Part print with two shaded views. Sizes in mm from the minimum x, y, z corner. Coordinates: 2 decimals unless noted, no trailing zeros. Write each loop counter-clockwise with the first axis right and the second up, starting at its lowest first coordinate (ties: lowest second). Pieces come first, ordered by that corner, then holes. Notation, with made-up numbers: (21, 86) - (77, 86) arc R5 cw to (77, 93) - close; hole circle Ø7 at (-27.5, -34). An arc over 180 degrees is marked (long way). Answer in a Markdown table with one row per item. Add a question column.
Q1. Band-saw the part on D-D (z = 20). List the corners of the cut face in (x, y).
Q2. Band-saw the part on C-C (x = 107.5). List the corners of the cut face in (y, z).
Q3. Drill centre lines: line 1 along Z through (x, y) = (205.25, 107.5); line 2 along Y through (x, z) = (104, 67.5). Where is each one in solid material? Low to high. Write a range as from..to.
Q4. Band-saw the part on A-A (y = 107.5). List the corners of the cut face in (x, z), and give its area (4 significant figures).
Q5. Band-saw the part on B-B (z = 106). List the corners of the cut face in (x, y).
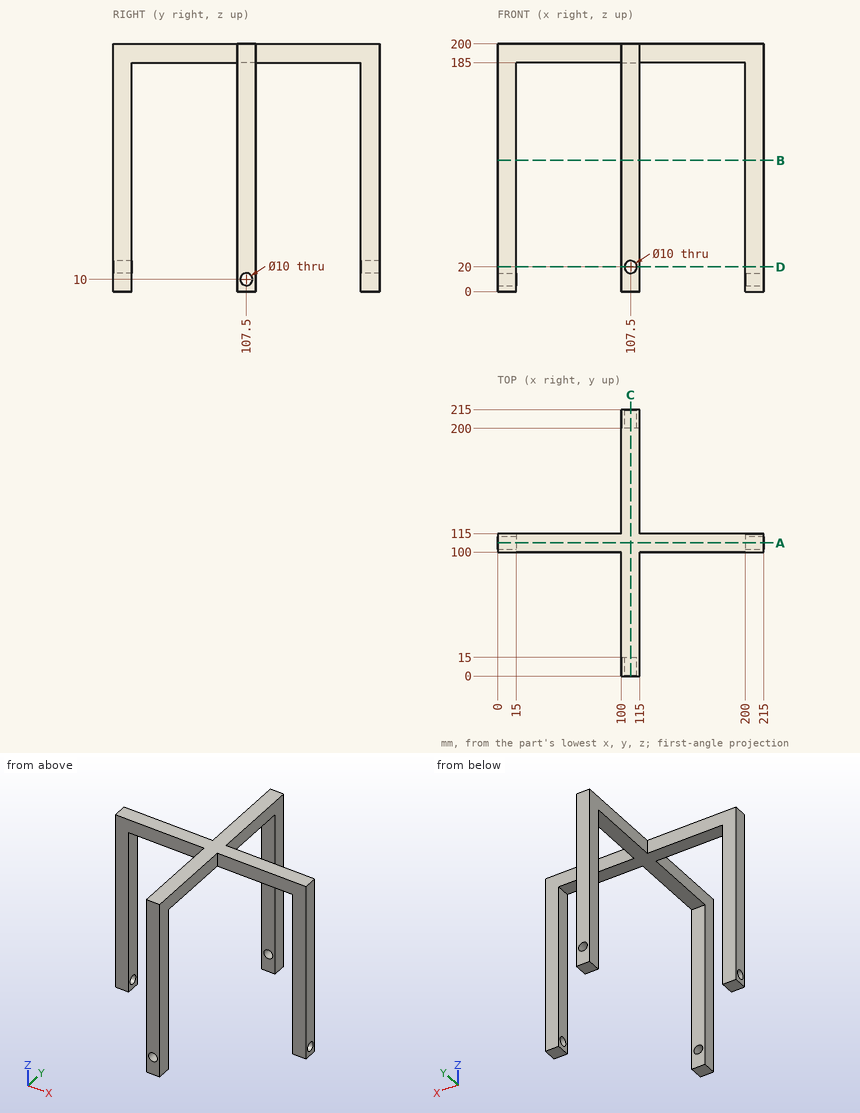
Checked values:
| question | item | result |
|---|---|---|
| 1 | outline | (0, 100) - (15, 100) - (15, 115) - (0, 115) - close; (100, 0) - (102.5, 0) - (102.5, 15) - (100, 15) - close; (100, 200) - (102.5, 200) - (102.5, 215) - (100, 215) - close; (112.5, 0) - (115, 0) - (115, 15) - (112.5, 15) - close; (112.5, 200) - (115, 200) - (115, 215) - (112.5, 215) - close; (200, 100) - (215, 100) - (215, 115) - (200, 115) - close |
| 2 | outline | (0, 0) - (15, 0) - (15, 15) - (0, 15) - close; (0, 25) - (15, 25) - (15, 185) - (200, 185) - (200, 25) - (215, 25) - (215, 200) - (0, 200) - close; (200, 0) - (215, 0) - (215, 15) - (200, 15) - close |
| 3 | line 1 | z = 0..5, 15..200 |
| 3 | line 2 | y = 0..15, 200..215 |
| 4 | outline | (0, 0) - (15, 0) - (15, 5) - (0, 5) - close; (0, 15) - (15, 15) - (15, 185) - (200, 185) - (200, 15) - (215, 15) - (215, 200) - (0, 200) - close; (200, 0) - (215, 0) - (215, 5) - (200, 5) - close |
| 4 | area | 8,475 mm² |
| 5 | outline | (0, 100) - (15, 100) - (15, 115) - (0, 115) - close; (100, 0) - (115, 0) - (115, 15) - (100, 15) - close; (100, 200) - (115, 200) - (115, 215) - (100, 215) - close; (200, 100) - (215, 100) - (215, 115) - (200, 115) - close |
